Verification items for the finished model (mm, model axes). A direction names the side the tool comes from. Round coordinates to 2 decimals unless told otherwise and drop trailing zeros. Order: outer loops, then holes, each group sorted by start corner. A loop starts at its lowest first (then second) coordinate and runs counter-clockwise, first axis right, second up. Notation, with made-up numbers: M 11,28 L 66,28 A15 ccw 66,55 Z; hole C 87.25,0.25 d3. An arc over 180 degrees is marked long. One line per item, written item: value. Start each with the question number.
from build123d import *

# Parameters (mm, degrees)
CROQUIS1_R              = 6.5
SALIENTE_EXTRUIR1_DEPTH = 23
CROQUIS2_R              = 3.95
SALIENTE_EXTRUIR2_DEPTH = 10
REDONDEO1_R             = 1
SALIENTE_EXTRUIR3_DEPTH = 6


with BuildPart() as part:
    # Croquis1 → Saliente-Extruir1 (new body)
    with BuildSketch(Plane.XY):
        Circle(CROQUIS1_R)
    extrude(amount=SALIENTE_EXTRUIR1_DEPTH)

    # Croquis2 → Saliente-Extruir2 (add)
    with BuildSketch(Plane.XY.offset(23)):
        Circle(CROQUIS2_R)
    extrude(amount=SALIENTE_EXTRUIR2_DEPTH)

    # Redondeo1
    redondeo1_edges = [part.edges().sort_by_distance(p)[0] for p in [
        (-3.95, 0, 23),
    ]]
    fillet(redondeo1_edges, radius=REDONDEO1_R)

    # Croquis3 → Saliente-Extruir3 (add)
    with BuildSketch(Plane(origin=(0, 0, 0), x_dir=(-1, 0, 0), z_dir=(0, 0, -1))):
        Polygon((-1.830695776, 5.775), (2.019304224, 5.775), (2.019304224, 1.925), (5.775, 1.925), (5.775, -1.925), (1.925, -1.925), (1.925, -5.775), (-1.925, -5.775), (-1.925, -1.925), (-5.680695776, -1.925), (-5.680695776, 1.925), (-1.830695776, 1.925), align=None)
    extrude(amount=SALIENTE_EXTRUIR3_DEPTH)


solid = part.part
1. Section check A-A (y = 0). Record the cut outline in (x, z) (3 decimals), and give its area (3 significant figures).
2. Depth check by flat-ended pin: pin 1 (3 mm diameter, centred on x = -1, y = 4, fed in from +Z); pin 2 (3 mm diameter, centred on y = -3, z = -3.5, fed in from +X); pin 3 (3 mm diameter, centred on x = 0.5, z = -3.5, fed in from -Y) (3 decimals); pin 4 (1.2 mm diameter, centred on y = 0, z = -2.5, fed in from -X) (3 decimals). Enter the tip coordinate at first touch or a pass-through.
3. Section check D-D (z = 27.5). Record the cut outline in (x, y).
4. Section check B-B (x = 0). Record the cut outline in (y, z) (3 decimals), and give its area (3 significant figures).
5. Section check C-C (z = -0.5). Record the cut outline in (x, y) (3 decimals).
6. Tool access check on faces 1 (the face through (1.831, 4, -3)), 2 (the face through (0, 5.775, -3)), 3 (the face through (-1.925, -4, -3)). Record the directions out of +Z, -Z, +X, -X, +Y, -Y that give a thin tool (end or side, any length) a straight path to the whole face; none if there is none.
7. Scan lines: line 1 along Z through (x, y) = (5, 1.25); line 2 along Y through (x, z) = (0, -2) (3 decimals); line 3 along Z through (x, y) = (-4.75, -3). Record each from-to range of solid material in increasing order.
Geometry check:
1. outline: M -6.5,0 L -5.775,0 L -5.775,-6 L 5.681,-6 L 5.681,0 L 6.5,0 L 6.5,23 L 4.95,23 A1 cw 3.95,24 L 3.95,33 L -3.95,33 L -3.95,24 A1 cw -4.95,23 L -6.5,23 Z
1. area: 447 mm²
2. pin 1: stops at z = 33
2. pin 2: stops at x = 5.68
2. pin 3: stops at y = -5.775
2. pin 4: stops at x = -5.775
3. outline: C 0,0 d7.9
4. outline: M -6.5,0 L -5.775,0 L -5.775,-6 L 5.775,-6 L 5.775,0 L 6.5,0 L 6.5,23 L 4.95,23 A1 cw 3.95,24 L 3.95,33 L -3.95,33 L -3.95,24 A1 cw -4.95,23 L -6.5,23 Z
4. area: 448 mm²
5. outline: M -5.775,-1.925 L -1.925,-1.925 L -1.925,-5.775 L 1.925,-5.775 L 1.925,-1.925 L 5.681,-1.925 L 5.681,1.925 L 1.831,1.925 L 1.831,5.775 L -2.019,5.775 L -2.019,1.925 L -5.775,1.925 Z
6. face 1: -Z, +X, +Y
6. face 2: -Z, +X, -X, +Y
6. face 3: -Z, -X, -Y
7. line 1: z = -6 to 23
7. line 2: y = -5.775 to 5.775
7. line 3: z = 0 to 23
